Can you work these out from the model? Positions are in its coordinate system, mm. Face numbers are marked on the shaded views. A direction names the side the tool comes from. Give positions to 0.01 mm unless a question says otherwise; leave off trailing zeros. Order: outer loops, then holes, each group sorted by start corner. A loop starts at its lowest first (then second) coordinate and runs counter-clockwise, first axis right, second up. Notation, with made-up numbers: (-21.5, 19) - (34.5, 19) arc R29 ccw to (34.5, 50) - close; hole circle Ø7 at (-20, 15.5). An arc over 180 degrees is marked (long way). Answer as a JSON object with one key per item and string values.
```python
from build123d import *

# Parameters (mm, degrees)
BOSS_EXTRUDE1_DEPTH = 12.7
SKETCH2_W           = 19.05
SKETCH2_H           = 6.35
CUT_EXTRUDE1_DEPTH  = 107.95
CUT_EXTRUDE2_DEPTH  = 64.816710194
CHAMFER1_SIZE       = 6.978592645
CHAMFER1_SIZE_2     = 2.54
CUT_EXTRUDE3_DEPTH  = 1.5875
CHAMFER3_SIZE       = 1.5875
FILLET1_R           = 6.35
FILLET2_R           = 1.27
FILLET3_R           = 5.08
CHAMFER4_SIZE       = 1.524


# Some blends are built 0.0001 mm under size
with BuildPart() as part:
    # Sketch1 → Boss-Extrude1 (new body)
    with BuildSketch(Plane(origin=(0, 0, 0), x_dir=(1, 0, 0), z_dir=(0, 1, 0))):
        with BuildLine():
            Line((-50.8, 12.7), (-57.15, 12.7))
            Line((-57.15, 12.7), (-57.15, 6.35))
            Line((-57.15, 6.35), (-57.15, -6.35))
            Line((-57.15, -6.35), (-57.15, -12.7))
            Line((-57.15, -12.7), (-50.8, -12.7))
            Line((-50.8, -12.7), (54.61, -12.7))
            ThreePointArc((54.61, -12.7), (56.406051224, -11.956051224), (57.15, -10.16))
            Line((57.15, -10.16), (57.15, 10.16))
            ThreePointArc((57.15, 10.16), (56.406051224, 11.956051224), (54.61, 12.7))
            Line((54.61, 12.7), (-50.8, 12.7))
        make_face()
    extrude(amount=BOSS_EXTRUDE1_DEPTH)

    # Sketch2 → Cut-Extrude1 (cut)
    with BuildSketch(Plane.ZY.offset(57.15)):
        with Locations((0, 9.525)):
            Rectangle(SKETCH2_W, SKETCH2_H)
    extrude(amount=-CUT_EXTRUDE1_DEPTH, mode=Mode.SUBTRACT)

    # Sketch3 → Cut-Extrude2 (cut, through all)
    with BuildSketch(Plane.XY.offset(12.7)):
        Polygon((25.4, 10.414), (57.15, 12.7), (-25.4, 12.7), (-19.05, 6.35), (50.8, 6.35), (50.8, 7.874), (27.15976362, 7.874), (25.4, 8.89), align=None)
    extrude(amount=-CUT_EXTRUDE2_DEPTH, mode=Mode.SUBTRACT)

    # Chamfer1
    # the kernel refuses this chamfer: 6.978592645, 2.54 mm, written as the material it adds along each edge
    with BuildSketch(Plane(origin=(-57.15, 6.35, 9.525), x_dir=(0, 0.9999130865277316, 0.013184058198642549), z_dir=(1, 0, 0))) as chamfer1_piece_1_section:
        Polygon((CHAMFER1_SIZE * 0.999913086587, -CHAMFER1_SIZE * 0.0131840581994), (-CHAMFER1_SIZE_2 * 0.0131840581987, -CHAMFER1_SIZE_2 * 0.999913086528), (0, 0), align=None)
    chamfer1_piece_1 = extrude(amount=56.203828281, mode=Mode.PRIVATE)
    chamfer1_piece_1 = split(chamfer1_piece_1, bisect_by=Plane(origin=(-39.199121236, 12.7, 8.706690515), z_dir=(0, -1, 0)), keep=Keep.TOP, mode=Mode.PRIVATE)
    chamfer1_piece_1 = split(chamfer1_piece_1, bisect_by=Plane(origin=(-30.223681853, 17.523681853, 8.706690515), z_dir=(-0.7071067811865448, -0.7071067811865503, 0)), keep=Keep.TOP, mode=Mode.PRIVATE)
    add(chamfer1_piece_1)
    with BuildSketch(Plane(origin=(-57.15, 6.35, -9.525), x_dir=(0, -0.09904090225207035, 0.9950833631817466), z_dir=(1, 0, 0))) as chamfer1_piece_2_section:
        Polygon((CHAMFER1_SIZE_2 * 0.995083363182, -CHAMFER1_SIZE_2 * 0.099040902252), (-CHAMFER1_SIZE * 0.099040902258, -CHAMFER1_SIZE * 0.995083363241), (0, 0), align=None)
    chamfer1_piece_2 = extrude(amount=56.203828281, mode=Mode.PRIVATE)
    chamfer1_piece_2 = split(chamfer1_piece_2, bisect_by=Plane(origin=(-30.223681853, 17.523681853, -8.706690515), z_dir=(-0.7071067811865448, -0.7071067811865503, 0)), keep=Keep.TOP, mode=Mode.PRIVATE)
    chamfer1_piece_2 = split(chamfer1_piece_2, bisect_by=Plane(origin=(-39.199121236, 12.7, -8.706690515), z_dir=(0, -1, 0)), keep=Keep.TOP, mode=Mode.PRIVATE)
    add(chamfer1_piece_2)

    # Sketch4 → Cut-Extrude3 (cut)
    with BuildSketch(Plane.XY.offset(12.7)):
        with BuildLine():
            Line((-57.15, 12.7), (-57.15, 0))
            Line((-57.15, 0), (-38.1, 0))
            Line((-38.1, 0), (-33.546051224, 4.553948776))
            ThreePointArc((-33.546051224, 4.553948776), (-32.802102448, 6.35), (-33.546051224, 8.146051224))
            Line((-33.546051224, 8.146051224), (-38.1, 12.7))
            Line((-38.1, 12.7), (-57.15, 12.7))
        make_face()
    cut_extrude3 = extrude(amount=-CUT_EXTRUDE3_DEPTH, mode=Mode.SUBTRACT)

    # Sketch6 → Cut-Revolve1 (revolve, cut)
    with BuildSketch(Plane.ZY.offset(40.64)):
        with BuildLine():
            Line((11.1125, 6.35), (11.1125, 11.43))
            ThreePointArc((11.1125, 11.43), (9.931118256, 9.01113492), (9.525, 6.35))
            Line((9.525, 6.35), (11.1125, 6.35))
        make_face()
    cut_revolve1 = revolve(axis=Axis((-40.64, 6.35, 12.7), (0, 0, -1)), mode=Mode.SUBTRACT)

    # Mirror1: Cut-Extrude3, Cut-Revolve1 across plane
    add(cut_extrude3.mirror(Plane(origin=(0, 0, 0), x_dir=(1, 0, 0), z_dir=(0, 0, -1))), mode=Mode.SUBTRACT)
    add(cut_revolve1.mirror(Plane(origin=(0, 0, 0), x_dir=(1, 0, 0), z_dir=(0, 0, -1))), mode=Mode.SUBTRACT)

    # Chamfer3
    chamfer3_edges = [part.edges().sort_by_distance(p)[0] for p in [
        (8.255, 0, 12.7),
        (56.406051224, 0, 11.956051224),
        (57.15, 0, 0),
        (56.406051224, 0, -11.956051224),
        (8.255, 0, -12.7),
    ]]
    chamfer(chamfer3_edges, length=CHAMFER3_SIZE)

    # Fillet1
    fillet1_edges = [part.edges().sort_by_distance(p)[0] for p in [
        (-57.15, 6.35, -11.1125),
        (-57.15, 6.35, 11.1125),
    ]]
    fillet(fillet1_edges, radius=FILLET1_R)

    # Fillet2
    fillet2_edges = [part.edges().sort_by_distance(p)[0] for p in [
        (-22.225, 9.525, 8.140605494),
        (-22.225, 9.525, -8.140605494),
        (25.4, 9.652, -9.525),
        (-22.225, 9.525, 12.7),
        (25.4, 9.652, 12.7),
        (25.4, 9.652, 9.525),
        (25.4, 9.652, -12.7),
        (-22.225, 9.525, -12.7),
    ]]
    fillet(fillet2_edges, radius=FILLET2_R)

    # Fillet3
    fillet3_edges = [part.edges().sort_by_distance(p)[0] for p in [
        (50.8, 10.0584, -9.525),
        (50.8, 10.0584, 9.525),
    ]]
    fillet(fillet3_edges, radius=FILLET3_R)

    # Chamfer4
    chamfer4_edges = [part.edges().sort_by_distance(p)[0] for p in [
        (50.8, 7.874, -8.5725),
        (50.8, 7.874, 8.5725),
    ]]
    chamfer(chamfer4_edges, length=CHAMFER4_SIZE - 0.0001)  # a hair under: the kernel refuses the full size


solid = part.part
```
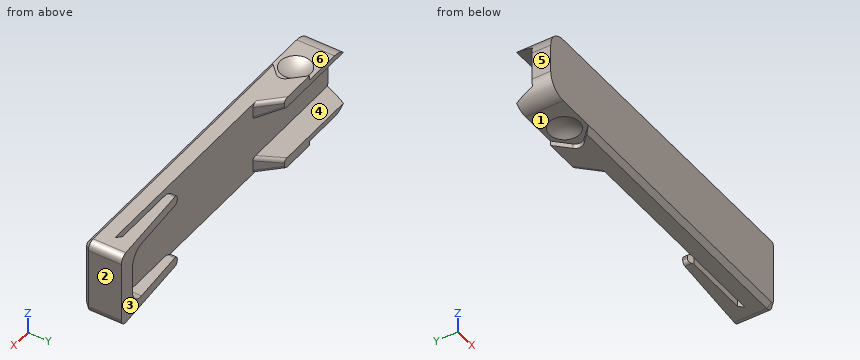
Q1. I need wall thicknesses on L1, parallel to X at y = 9, z = 4.5; L2, parallel to Y at x = 34, z = -5.75. Which ranges of each line are inside material? Lowest first, please.
Recorded:
{"L1": "x = 50.8 to 57.15", "L2": "y = 0 to 6.35"}
Q2. If we section it at C-C, the plane x = -16: Please give me the cut outline in (y, z), then the cut area to 3 significant figures.
Recorded:
{"outline": "(0, -11.11) - (1.59, -12.7) - (6.35, -12.7) - (6.35, 12.7) - (1.59, 12.7) - (0, 11.11) - close", "area": "159 mm^2"}
Q3. If we section it at A-A, the plane z = 0: Please give me the cut outline in (x, y).
Recorded:
{"outline": "(-57.15, 0) - (55.56, 0) - (57.15, 1.59) - (57.15, 12.7) - (50.8, 12.24) - (50.8, 6.35) - (-57.15, 6.35) - close"}
Q4. I'm going to push flat-ended pins straight in: pin 1 Ø5 at (x, y) = (21, 10.5) entering from -Z; pin 2 Ø6 at (x, y) = (-11.5, 6.5) entering from +Z; pin 3 Ø2 at (y, z) = (6, -6) entering from -X; pin 4 Ø3 at (y, z) = (9, -0.5) entering from -X. Where does each tip first touch, or does it pass through?
Recorded:
{"pin 1": "passes through", "pin 2": "stops at z = 12.7", "pin 3": "stops at x = -57.15", "pin 4": "stops at x = 50.8"}
Q5. Which directions (+Z, -Z, +X, -X, +Y, -Y) give clear straight access to the entire face, cutting with the end or side of a thin tool? Please do the marked faces 4, 5 and 6.
Recorded:
{"face 4": "-X, +Y", "face 5": "+Z, -Z, -X, +Y, -Y", "face 6": "+Z, -X"}
Q6. If we section it at B-B, the plane y = 3: Please give me the cut outline in (x, z), then the cut area to 3 significant figures.
Recorded:
{"outline": "(-57.15, -4.76) arc R6.35 ccw to (-50.8, -11.11) - (-44.46, -11.11) arc R8.27 cw to (-36.82, -11.11) - (-35.1, -11.11) - (-35.1, -12.7) - (54.61, -12.7) arc R2.54 ccw to (57.15, -10.16) - (57.15, 10.16) arc R2.54 ccw to (54.61, 12.7) - (-35.1, 12.7) - (-35.1, 11.11) - (-36.82, 11.11) arc R8.27 cw to (-44.46, 11.11) - (-50.8, 11.11) arc R6.35 ccw to (-57.15, 4.76) - close", "area": "2,800 mm^2"}
Q7. We'd pull the mould along Y, two halves only. Please class the marked faces 1, 2 and 3: released by +Y, released by -Y, zero draft, split by the parting line, or undercut.
Recorded:
{"face 1": "undercut", "face 2": "zero draft", "face 3": "released by +Y"}
